from build123d import *

# Parameters (mm, degrees)
SKETCH1_W           = 800
SKETCH1_H           = 800
BOSS_EXTRUDE1_DEPTH = 100
SKETCH2_R           = 250
SKETCH2_R_2         = 200
BOSS_EXTRUDE2_DEPTH = 1000
FILLET1_R           = 20


with BuildPart() as part:
    # Sketch1 → Boss-Extrude1 (new body)
    with BuildSketch(Plane.XY):
        Rectangle(SKETCH1_W, SKETCH1_H)
    extrude(amount=BOSS_EXTRUDE1_DEPTH)

    # Sketch2 → Boss-Extrude2 (add)
    with BuildSketch(Plane.XY.offset(100)):
        with Locations(Location((0, 0, 0), (0, 0, 180))):
            Circle(SKETCH2_R)
        Circle(SKETCH2_R_2, mode=Mode.SUBTRACT)
    extrude(amount=BOSS_EXTRUDE2_DEPTH)

    # Fillet1
    fillet1_edges = [part.edges().sort_by_distance(p)[0] for p in [
        (-400, 0, 100),
        (0, -400, 100),
        (400, 0, 100),
        (0, 400, 100),
    ]]
    fillet(fillet1_edges, radius=FILLET1_R)


solid = part.part
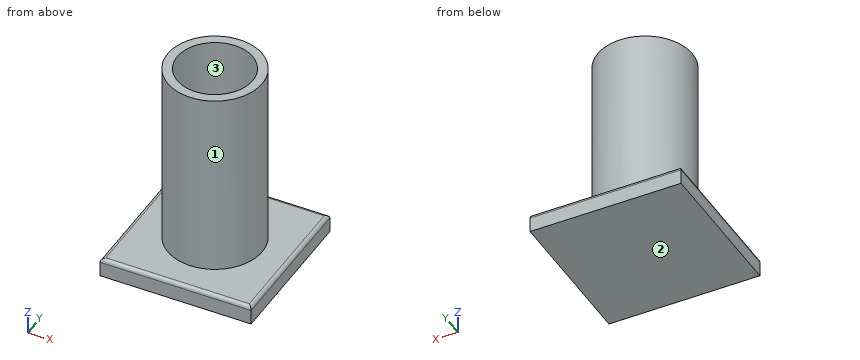
The model under review builds one solid part; all positions refer to its coordinate system, in mm. Face numbers are marked on the shaded views. Give positions to 0.01 mm unless a question says otherwise; leave off trailing zeros. Order: outer loops, then holes, each group sorted by start corner. A loop starts at its lowest first (then second) coordinate and runs counter-clockwise, first axis right, second up. Notation, with made-up numbers: (6, -0.75) -> (29, -0.75) arc R31 cw to (29, 37.25) -> close; hole circle Ø1 at (62, 76.5). An arc over 180 degrees is marked (long way). Write item = value, one per line. Start each with the question number.
(1) For L1, parallel to Y at x = 0, z = 855; L2, parallel to Y at x = 7, z = 863.5; L3, parallel to Z at x = 38, y = -293.5, list the stretches that pass through material, from the lowest coordinate up. Write a range as from..to.
(2) Draft analysis for pull direction X (two halves, no side actions). For the marked faces 1, 2 and 3, state which applies: +X half, -X half, draft (parallel to the pull), parting line (faces both ways), or undercut.
(3) Take a section at C-C (z = 396). Write out the cut boundary in (x, y).
(4) Take a section at D-D (y = 332). Write out the cut boundary in (x, z), plus the area to 3 significant figures.
(5) For pin 1 Ø10 at (y, z) = (-136, 475) entering from +X; pin 2 Ø1 at (x, z) = (-79, 263.5) entering from -Y; pin 3 Ø1.5 at (y, z) = (178.5, 207.5) entering from -X, all flat-tipped, find the tip position at first contact; note any pin that passes through.
(6) Take a section at A-A (y = 0). Write out the cut boundary in (x, z), plus the area to 3 significant figures.
Returned:
q1.L1 = -250..-200, 200..250
q1.L2 = -249.9..-199.88, 199.88..249.9
q1.L3 = 0..100
q2.face_1 = parting line
q2.face_2 = draft
q2.face_3 = undercut
q3.outline = circle Ø500 at (0, 0); hole circle Ø400 at (0, 0)
q4.outline = (-400, 0) -> (400, 0) -> (400, 80) arc R20 ccw to (380, 100) -> (-380, 100) arc R20 ccw to (-400, 80) -> close
q4.area = 79,800 mm²
q5.pin_1 = 212.93
q5.pin_2 = -237.36
q5.pin_3 = -175.8
q6.outline = (-400, 0) -> (400, 0) -> (400, 80) arc R20 ccw to (380, 100) -> (250, 100) -> (250, 1100) -> (200, 1100) -> (200, 100) -> (-200, 100) -> (-200, 1100) -> (-250, 1100) -> (-250, 100) -> (-380, 100) arc R20 ccw to (-400, 80) -> close
q6.area = 180,000 mm²
